Build history of the part. All positions in model axes, mm. A direction names the side the tool comes from. Give positions to 0.01 mm unless a question says otherwise; leave off trailing zeros. Loops run counter-clockwise (first coordinate to the right, second up) from the corner with the lowest first, then second, coordinate; pieces in that order, holes last. Notation, with made-up numbers: (44, 38.25) -> (52, 38.25) arc R17 ccw to (52, 46.25) -> close; hole circle Ø10 at (-32.75, -19.75). An arc over 180 degrees is marked (long way). Answer as a JSON object with one key per item and string values. Group by question number.
from build123d import *

# Parameters (mm, degrees)
BOSS_EXTRUDE1_DEPTH  = 9.6
CHAMFER2_SIZE        = 0.6
CUT_EXTRUDE2_DEPTH   = 2.5
M2_CLEARANCE_HOLE1_D = 2.6
CUT_EXTRUDE3_START   = -9.6
CUT_EXTRUDE3_DEPTH   = 5.5


with BuildPart() as part:
    # Sketch1 → Boss-Extrude1 (new body)
    with BuildSketch(Plane.XY):
        with BuildLine():
            ThreePointArc((-11.756599923, -15.949743136), (-6.144180323, -14.833363466), (-2.965, -19.591343059))
            Line((-2.965, -19.591343059), (2.965, -19.591343059))
            ThreePointArc((2.965, -19.591343059), (6.144180323, -14.833363466), (11.756599923, -15.949743136))
            Line((11.756599923, -15.949743136), (15.949743136, -11.756599923))
            ThreePointArc((15.949743136, -11.756599923), (14.833363466, -6.144180323), (19.591343059, -2.965))
            Line((19.591343059, -2.965), (19.591343059, 2.965))
            ThreePointArc((19.591343059, 2.965), (14.833363466, 6.144180323), (15.949743136, 11.756599923))
            Line((15.949743136, 11.756599923), (11.756599923, 15.949743136))
            ThreePointArc((11.756599923, 15.949743136), (6.144180323, 14.833363466), (2.965, 19.591343059))
            Line((2.965, 19.591343059), (-2.965, 19.591343059))
            ThreePointArc((-2.965, 19.591343059), (-6.144180323, 14.833363466), (-11.756599923, 15.949743136))
            Line((-11.756599923, 15.949743136), (-15.949743136, 11.756599923))
            ThreePointArc((-15.949743136, 11.756599923), (-14.833363466, 6.144180323), (-19.591343059, 2.965))
            Line((-19.591343059, 2.965), (-19.591343059, -2.965))
            ThreePointArc((-19.591343059, -2.965), (-14.833363466, -6.144180323), (-15.949743136, -11.756599923))
            Line((-15.949743136, -11.756599923), (-11.756599923, -15.949743136))
        make_face()
    extrude(amount=BOSS_EXTRUDE1_DEPTH)

    # Chamfer2
    chamfer2_edges = [part.edges().sort_by_distance(p)[0] for p in [
        (-19.591343059, 0, 9.6),
        (-13.853171529, 13.853171529, 0),
        (0, 19.591343059, 0),
        (13.853171529, 13.853171529, 0),
        (19.591343059, 0, 0),
        (-13.853171529, -13.853171529, 9.6),
        (13.853171529, -13.853171529, 0),
        (0, -19.591343059, 0),
        (-13.853171529, -13.853171529, 0),
        (-19.591343059, 0, 0),
        (0, -19.591343059, 9.6),
        (13.853171529, -13.853171529, 9.6),
        (19.591343059, 0, 9.6),
        (13.853171529, 13.853171529, 9.6),
        (0, 19.591343059, 9.6),
        (-13.853171529, 13.853171529, 9.6),
    ]]
    chamfer(chamfer2_edges, length=CHAMFER2_SIZE)

    # Sketch4 → Cut-Extrude2 (cut)
    with BuildSketch(Plane.XY.offset(9.6)):
        with BuildLine():
            ThreePointArc((14.441692106, -1.95061736), (16, 0), (14.441692106, 1.95061736))
            Line((14.441692106, 1.95061736), (6.69085075, 3.70569527))
            Line((6.69085075, 3.70569527), (6.495190528, 3.75))
            Line((6.495190528, 3.75), (6.554651618, 3.941599088))
            Line((6.554651618, 3.941599088), (6.750311839, 3.897294358))
            Line((6.750311839, 3.897294358), (9.101143263, 11.472284348))
            ThreePointArc((9.101143263, 11.472284348), (8.1, 14.029611541), (5.384718053, 13.617963443))
            Line((5.384718053, 13.617963443), (0, 7.794588715))
            Line((0, 7.794588715), (-5.384718053, 13.617963443))
            ThreePointArc((-5.384718053, 13.617963443), (-8.1, 14.029611541), (-9.101143263, 11.472284348))
            Line((-9.101143263, 11.472284348), (-6.750311839, 3.897294358))
            Line((-6.750311839, 3.897294358), (-14.485861316, 2.145679096))
            ThreePointArc((-14.485861316, 2.145679096), (-16.2, 0), (-14.485861316, -2.145679096))
            Line((-14.485861316, -2.145679096), (-6.750311839, -3.897294358))
            Line((-6.750311839, -3.897294358), (-9.101143263, -11.472284348))
            ThreePointArc((-9.101143263, -11.472284348), (-8.1, -14.029611541), (-5.384718053, -13.617963443))
            Line((-5.384718053, -13.617963443), (0, -7.794588715))
            Line((0, -7.794588715), (5.384718053, -13.617963443))
            ThreePointArc((5.384718053, -13.617963443), (8.1, -14.029611541), (9.101143263, -11.472284348))
            Line((9.101143263, -11.472284348), (6.750311839, -3.897294358))
            Line((6.750311839, -3.897294358), (6.554651618, -3.941599088))
            Line((6.554651618, -3.941599088), (6.495190528, -3.75))
            Line((6.495190528, -3.75), (6.69085075, -3.70569527))
            Line((6.69085075, -3.70569527), (14.441692106, -1.95061736))
        make_face()
    extrude(amount=-CUT_EXTRUDE2_DEPTH, mode=Mode.SUBTRACT)

    # M2 Clearance Hole1 (through all)
    with Locations(Plane.XY.offset(7.1)):
        with Locations((13.5, 0), (6.75, -11.691342951), (-6.75, -11.691342951), (-13.5, 0), (-6.75, 11.691342951), (6.75, 11.691342951)):
            Hole(M2_CLEARANCE_HOLE1_D / 2)

    # Sketch3<2> → Cut-Extrude3 (cut)
    with BuildSketch(Plane.XY.offset(9.6).offset(CUT_EXTRUDE3_START)):
        with BuildLine():
            Line((-2, -1.5), (-5.5, -1.5))
            Line((-5.5, -1.5), (-5.5, 1.5))
            Line((-5.5, 1.5), (-2, 1.5))
            ThreePointArc((-2, 1.5), (0, 2.5), (2, 1.5))
            Line((2, 1.5), (5.5, 1.5))
            Line((5.5, 1.5), (5.5, -1.5))
            Line((5.5, -1.5), (2, -1.5))
            ThreePointArc((2, -1.5), (0, -2.5), (-2, -1.5))
        make_face()
    extrude(amount=CUT_EXTRUDE3_DEPTH, mode=Mode.SUBTRACT)


solid = part.part
(1) Saw through at C-C on x = 13.5. List the corners of the cut face in (y, z).
(2) Saw through at A-A on x = -13.5. List the corners of the cut face in (y, z).
(3) Saw through at D-D on x = 1.5. List the corners of the cut face in (y, z).
(4) Probe line 1 along Y through (x, z) = (2.5, 4.75); line 2 along Y through (x, z) = (6, 2); line 3 along Y through (x, z) = (-6.75, 3). List the from-to ranges inside material, lowest first. Write a range as [from, to].
(5) Pin check, flat tips, straight feed: pin 1 (1 mm diameter, centred on y = -14, z = 2, fed in from +X); pin 2 (1 mm diameter, centred on x = -14, z = 6.5, fed in from +Y); pin 3 (1 mm diameter, centred on x = -4.5, z = 3, fed in from +Y). Stop position of each tip, or through.
(6) 3-axis set-ups, long thin cutter, end or side, ignore diameter. For faces 4 (the flat face through (7.9, 7.6, 8.4)), 5 (the flat face through (0, 0, 5.5)), 6 (the cylindrical face through (-6.066, 14.867, 4.733)): which of +Z, -Z, +X, -X, +Y, -Y reach the whole face in a straight line?
(7) Pull direction Y, two halves, no side cores. Call faces 1 (the flat face through (13.824, -13.883, 4.741)), 2 (the flat face through (-13.824, 13.883, 4.741)), 3 (the cylindrical face through (-14.867, -6.066, 4.733)): pulls with the +Y half, pulls with the -Y half, needs draft (parallel to the pull), parting line crosses it, or undercut.
(8) Saw through at B-B on z = 6. List the corners of the cut face in (x, y) (3 decimals), plus the area to 3 significant figures.
Calculated:
{
 "1": {"outline": "(-14.21, 0.6) -> (-13.36, 0) -> (-1.3, 0) -> (-1.3, 7.1) -> (-2.16, 7.1) -> (-2.16, 9.6) -> (-13.36, 9.6) -> (-14.21, 9) -> close; (1.3, 0) -> (13.36, 0) -> (14.21, 0.6) -> (14.21, 9) -> (13.36, 9.6) -> (2.16, 9.6) -> (2.16, 7.1) -> (1.3, 7.1) -> close"},
 "2": {"outline": "(-14.21, 0.6) -> (-13.36, 0) -> (-1.3, 0) -> (-1.3, 7.1) -> (-2.37, 7.1) -> (-2.37, 9.6) -> (-13.36, 9.6) -> (-14.21, 9) -> close; (1.3, 0) -> (13.36, 0) -> (14.21, 0.6) -> (14.21, 9) -> (13.36, 9.6) -> (2.37, 9.6) -> (2.37, 7.1) -> (1.3, 7.1) -> close"},
 "3": {"outline": "(-19.59, 0.6) -> (-18.99, 0) -> (-2, 0) -> (-2, 5.5) -> (2, 5.5) -> (2, 0) -> (18.99, 0) -> (19.59, 0.6) -> (19.59, 9) -> (18.99, 9.6) -> (9.42, 9.6) -> (9.42, 7.1) -> (-9.42, 7.1) -> (-9.42, 9.6) -> (-18.99, 9.6) -> (-19.59, 9) -> close"},
 "4": {"line 1": "y = [-19.59, -1.5], [1.5, 19.59]", "line 2": "y = [-14.9, -12.75], [-10.63, 10.63], [12.75, 14.9]", "line 3": "y = [-14.63, -12.99], [-10.39, 10.39], [12.99, 14.63]"},
 "5": {"pin 1": "stops at x = 14.21", "pin 2": "stops at y = 14.21", "pin 3": "stops at y = 16.49"},
 "6": {"face 4": "+Z", "face 5": "-Z", "face 6": "+Z, -Z, +Y"},
 "7": {"face 1": "pulls with the -Y half", "face 2": "pulls with the +Y half", "face 3": "undercut"},
 "8": {"outline": "(-19.591, -2.965) arc R5.15 cw to (-15.95, -11.757) -> (-11.757, -15.95) arc R5.15 cw to (-2.965, -19.591) -> (2.965, -19.591) arc R5.15 cw to (11.757, -15.95) -> (15.95, -11.757) arc R5.15 cw to (19.591, -2.965) -> (19.591, 2.965) arc R5.15 cw to (15.95, 11.757) -> (11.757, 15.95) arc R5.15 cw to (2.965, 19.591) -> (-2.965, 19.591) arc R5.15 cw to (-11.757, 15.95) -> (-15.95, 11.757) arc R5.15 cw to (-19.591, 2.965) -> close; hole circle Ø2.6 at (-13.5, 0); hole circle Ø2.6 at (-6.75, -11.691); hole circle Ø2.6 at (-6.75, 11.691); hole circle Ø2.6 at (6.75, -11.691); hole circle Ø2.6 at (6.75, 11.691); hole circle Ø2.6 at (13.5, 0)", "area": "990 mm^2"}
}
